Model file for the job. Use its own axes, mm. A direction names the side the tool comes from. Coordinates: 2 decimals unless noted, no trailing zeros. Write each loop counter-clockwise with the first axis right and the second up, starting at its lowest first coordinate (ties: lowest second). Pieces come first, ordered by that corner, then holes. Notation, with made-up numbers: (8.25, -26) - (39.25, -26) arc R15 ccw to (39.25, -7) - close; hole circle Ø4 at (66.25, 49.5). An arc over 180 degrees is marked (long way). Put each result on its own line as item: value. Start each with the question number.
1. Drill centre lines: L1, parallel to Y at x = -24, z = 73.5 (3 decimals); L2, parallel to Y at x = -19.5, z = 22. Where is each one in solid material? Low to high. Write a range as from..to.
2. Pull direction X, two halves, no side cores. Call faces 1 (the face through (0, -10.77, 54)), 2 (the face through (21.36, 8.305, 55.516)), 3 (the face through (7, -5.77, 5)), 4 (the face through (7, -5.77, 85)): released by +X, released by -X, zero draft, split by the parting line, or undercut.
3. Which spindle directions (+Z, -Z, +X, -X, +Y, -Y) get a long thin tool onto all of the face, cutting with end or side? Do faces 5 (the face through (0, 0, 0)), 6 (the face through (7, -8, 86)). Say none if no direction does.
4. Saw through at C-C, the plane x = 28. Write the cut outline in (y, z) (3 decimals), plus the area to 3 significant figures.
5. Drop flat-ended pins along their axis: P1, Ø6, axis at x = 18.5, z = 59.5, coming from the +Y side; P2, Ø1.2, axis at x = 7, z = 5, coming from the -Y side. Give the stop position or say it passes through.
6. Saw through at B-B, the plane x = -20.5. Write the cut outline in (y, z), plus the area to 3 significant figures.
7. Saw through at A-A, the plane z = 52. Write the cut outline in (x, y), plus the area to 3 significant figures.
```python
from build123d import *

# Parameters (mm, degrees)
SKETCH_1_W          = 63
SKETCH_1_H          = 21.54
EXTRUDE_1_DEPTH     = 109.5
CUT_EXTRUDE_1_DEPTH = 115.448647436
SKETCH_3_R          = 1
CUT_EXTRUDE_2_DEPTH = 5


with BuildPart() as part:
    # 草图1 → 凸台-拉伸1 (new body)
    with BuildSketch(Plane.XY):
        Rectangle(SKETCH_1_W, SKETCH_1_H)
    extrude(amount=EXTRUDE_1_DEPTH)

    # 草图2 → 切除-拉伸1 (cut, through all)
    with BuildSketch(Plane.XY.offset(109.5)):
        Polygon((11.5, 10.77), (31.5, 5.77), (31.5, 10.77), align=None)
        Polygon((-31.5, 10.77), (-11.5, 10.77), (-31.5, 5.77), align=None)
        Polygon((-31.5, -8.77), (-11.5, -10.77), (-31.5, -10.77), align=None)
        Polygon((31.5, -8.77), (11.5, -10.77), (31.5, -10.77), align=None)
    extrude(amount=-CUT_EXTRUDE_1_DEPTH, mode=Mode.SUBTRACT)

    # 草图3 → 切除-拉伸2 (cut)
    with BuildSketch(Plane.XZ.offset(10.77)):
        with Locations(Location((-7, 5, 0), (0, 0, 270))):
            Circle(SKETCH_3_R)
        with Locations(Location((7, 5, 0), (0, 0, 270))):
            Circle(SKETCH_3_R)
        with Locations(Location((-7, 85, 0), (0, 0, 270))):
            Circle(SKETCH_3_R)
        with Locations(Location((7, 85, 0), (0, 0, 270))):
            Circle(SKETCH_3_R)
    extrude(amount=-CUT_EXTRUDE_2_DEPTH, mode=Mode.SUBTRACT)


solid = part.part
```
Final values:
1. L1: y = -9.52..7.645
1. L2: y = -9.97..8.77
2. face 1: zero draft
2. face 2: released by +X
2. face 3: undercut
2. face 4: undercut
3. face 5: -Z, +X, -X, +Y, -Y
3. face 6: -Y
4. outline: (-9.12, 0) - (6.645, 0) - (6.645, 109.5) - (-9.12, 109.5) - close
4. area: 1,730 mm²
5. P1: stops at y = 9.77
5. P2: stops at y = -5.77
6. outline: (-9.87, 0) - (8.52, 0) - (8.52, 109.5) - (-9.87, 109.5) - close
6. area: 2,010 mm²
7. outline: (-31.5, -8.77) - (-11.5, -10.77) - (11.5, -10.77) - (31.5, -8.77) - (31.5, 5.77) - (11.5, 10.77) - (-11.5, 10.77) - (-31.5, 5.77) - close
7. area: 1,220 mm²
